Work out the finished part from the listing and answer in its coordinate system (mm). Face numbers are marked on the shaded views. A direction names the side the tool comes from. Coordinates: 2 decimals unless noted, no trailing zeros. Order: outer loops, then holes, each group sorted by start corner. A loop starts at its lowest first (then second) coordinate and runs counter-clockwise, first axis right, second up. Notation, with made-up numbers: (85, 4) -> (99, 4) arc R19 ccw to (99, 15) -> close; hole circle Ø7 at (-20.75, 61.25). An arc over 180 degrees is marked (long way). Write item = value, one per line. Start each with the question number.
Q1. Which of the six approach directions +Z, -Z, +X, -X, +Y, -Y give full straight-line access (tool end or side, diameter ignored) to the marked faces 1, 2 and 3?
Q2. For a pull along Z with two mould halves and no side action, classify the marked faces 4, 5 and 6 as +Z half, -Z half, draft (parallel to the pull), parting line (faces both ways), or undercut.
Q3. The part is cut by section D-D, the plane y = 7. Count the separate pieces of the cut face and the enclosed holes in it, plus the area to 3 significant figures.
Q4. The part is cut by section B-B, the plane z = -40. Determine the outline of the cut face in (x, y), plus the area to 3 significant figures.
Q5. The part is cut by section A-A, the plane y = 20. Determine the outline of the cut face in (x, z).
Q6. Flat-ended cylindrical pins translate along their axes: pin 1 (8 mm diameter, centred on y = 9, z = -114, fed in from -X); pin 2 (1 mm diameter, centred on x = -19, y = 29.5, fed in from -Z); pin 3 (13 mm diameter, centred on y = 9.5, z = -116, fed in from +X). Find the tip coordinate at first contact, or state that the pin passes through.
Q7. Straight lines are drawn through the part: L1, parallel to Z at x = 0, y = 12; L2, parallel to Y at x = 12, z = -77; L3, parallel to Z at x = -4, y = 57. For each, find the intervals that lie inside material, in ascending order. Write a range as from..to.
Q8. The part is cut by section C-C, the plane x = -21. Determine the outline of the cut face in (y, z).
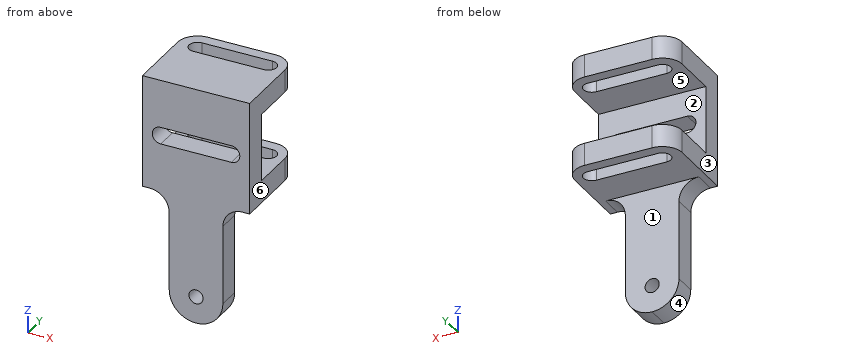
```python
from build123d import *

# Parameters (mm, degrees)
ESTRUSIONE_ESTRUSIONE1_DEPTH = 38
SCHIZZO3_W                   = 38
SCHIZZO3_H                   = 89
ESTRUSIONE_ESTRUSIONE2_DEPTH = 16
RACCORDO1_R                  = 19
RACCORDO2_R                  = 14
TAGLIO_ESTRUSIONE1_REACH     = 181.223
TAGLIO_ESTRUSIONE2_DEPTH     = 184.980977278
FORO_10_0_10_2_D             = 10
RACCORDO3_R                  = 14


with BuildPart() as part:
    # Schizzo2 → Estrusione-Estrusione1 (new, symmetric)
    with BuildSketch(Plane(origin=(0, 0, 0), x_dir=(0, 0, -1), z_dir=(1, 0, 0))):
        Polygon((0, 62), (0, 0), (80, 0), (80, 62), (64, 62), (64, 16), (16, 16), (16, 62), align=None)
    extrude(amount=ESTRUSIONE_ESTRUSIONE1_DEPTH, both=True)

    # Schizzo3 → Estrusione-Estrusione2 (add)
    with BuildSketch(Plane.XZ):
        with Locations((0, -124.5)):
            Rectangle(SCHIZZO3_W, SCHIZZO3_H)
    extrude(amount=-ESTRUSIONE_ESTRUSIONE2_DEPTH)

    # Raccordo1
    raccordo1_edges = [part.edges().sort_by_distance(p)[0] for p in [
        (19, 8, -169),
        (-19, 8, -169),
    ]]
    fillet(raccordo1_edges, radius=RACCORDO1_R - 0.0001)  # a hair under: the kernel refuses the full size

    # Raccordo2
    raccordo2_edges = [part.edges().sort_by_distance(p)[0] for p in [
        (-38, 62, -8),
        (38, 62, -72),
        (38, 62, -8),
        (-38, 62, -72),
    ]]
    fillet(raccordo2_edges, radius=RACCORDO2_R)

    # Schizzo4 → Taglio-Estrusione1 (cut, up to next)
    with BuildSketch(Plane(origin=(0, 16, 0), x_dir=(1, 0, 0), z_dir=(0, 1, 0)), mode=Mode.PRIVATE) as taglio_estrusione1_sk1:
        with BuildLine():
            Line((25, 34), (-25, 34))
            ThreePointArc((-25, 34), (-31, 40), (-25, 46))
            Line((-25, 46), (25, 46))
            ThreePointArc((25, 46), (31, 40), (25, 34))
        make_face()
    taglio_estrusione1_tool1 = extrude(taglio_estrusione1_sk1.sketch, amount=-TAGLIO_ESTRUSIONE1_REACH, mode=Mode.PRIVATE) & part.part
    add(taglio_estrusione1_tool1.solids().sort_by_distance((0, 16, -40))[0], mode=Mode.SUBTRACT)

    # Schizzo5 → Taglio-Estrusione2 (cut, through all)
    with BuildSketch(Plane.XY):
        with BuildLine():
            Line((-24, 54), (26, 54))
            ThreePointArc((26, 54), (32, 48), (26, 42))
            Line((26, 42), (-24, 42))
            ThreePointArc((-24, 42), (-30, 48), (-24, 54))
        make_face()
    extrude(amount=-TAGLIO_ESTRUSIONE2_DEPTH, mode=Mode.SUBTRACT)

    # Foro Ø10.0 (10)-2 (through all)
    with Locations(Plane(origin=(0, 16, 0), x_dir=(1, 0, 0), z_dir=(0, 1, 0))):
        with Locations((0, 150)):
            Hole(FORO_10_0_10_2_D / 2)

    # Raccordo3
    raccordo3_edges = [part.edges().sort_by_distance(p)[0] for p in [
        (-19, 8, -80),
        (19, 8, -80),
    ]]
    fillet(raccordo3_edges, radius=RACCORDO3_R)


solid = part.part
```
Model answer:
q1.face_1 = -Z, +X, -X, +Y
q1.face_2 = +X, -X, +Y
q1.face_3 = +Z, -Z, -X, +Y, -Y
q2.face_4 = -Z half
q2.face_5 = undercut
q2.face_6 = draft
q3.separate_pieces = 1
q3.enclosed_holes = 2
q3.area = 8,600 mm2
q4.outline = (-38, 0) -> (-31, 0) -> (-31, 16) -> (-38, 16) -> close; (31, 0) -> (38, 0) -> (38, 16) -> (31, 16) -> close
q4.area = 224 mm2
q5.outline = (-38, -80) -> (38, -80) -> (38, -64) -> (-38, -64) -> close; (-38, -16) -> (38, -16) -> (38, 0) -> (-38, 0) -> close
q6.pin_1 = -19
q6.pin_2 = -80
q6.pin_3 = 19
q7.L1 = -169..-155, -145..-46, -34..0
q7.L2 = 0..42, 54..62
q7.L3 = -80..-64, -16..0
q8.outline = (0, -86.79) -> (16, -86.79) -> (16, -80) -> (42, -80) -> (42, -64) -> (16, -64) -> (16, -46) -> (0, -46) -> close; (0, -34) -> (16, -34) -> (16, -16) -> (42, -16) -> (42, 0) -> (0, 0) -> close; (54, -80) -> (62, -80) -> (62, -64) -> (54, -64) -> close; (54, -16) -> (62, -16) -> (62, 0) -> (54, 0) -> close
